from build123d import *

# Parameters (mm, degrees)
EXTRUDE_1_DEPTH = 20


with BuildPart() as part:
    # Эскиз1 → Бобышка-Вытянуть1 (new body)
    with BuildSketch(Plane.XY):
        Polygon((-9.845304567, -8.192930284), (40.154695433, -8.192930284), (40.154695433, -2.192930284), (19.154695433, -2.192930284), (19.154695433, -0.692930284), (23.154695433, 1.307069716), (23.154695433, 2.307069716), (19.154695433, 4.307069716), (11.154695433, 4.307069716), (7.154695433, 2.307069716), (7.154695433, 1.307069716), (11.154695433, -0.692930284), (11.154695433, -2.192930284), (-9.845304567, -2.192930284), align=None)
    extrude(amount=EXTRUDE_1_DEPTH)


solid = part.part
Read the model definition and answer for the solid it produces. Units are mm, in the model's axes. A direction names the side the tool comes from. Round coordinates to 2 decimals unless told otherwise and drop trailing zeros. Write each loop counter-clockwise with the first axis right and the second up, starting at its lowest first coordinate (ties: lowest second). Pieces come first, ordered by that corner, then holes.
1. Given pin 1 Ø1.2 at (y, z) = (-1.5, 10.5) entering from -X; pin 2 Ø6 at (x, z) = (28, 8) entering from +Y; pin 3 Ø0.8 at (y, z) = (1.5, 7.5) entering from -X; pin 4 Ø1.5 at (x, y) = (33, -4.5) entering from -Z, each flat-ended and moving along its own axis, determine where each tip first touches the part or whether it passes through.
2. Determine the mould class of faces 5 (the face through (19.155, -1, 10)), 6 (the face through (15, -8.193, 10)), 7 (the face through (21.127, 0.293, 9.86)), 8 (the face through (15, -3, 20)) for opening direction Y: pulls with the +Y half, pulls with the -Y half, needs draft (parallel to the pull), parting line crosses it, or undercut.
3. The part is cut by section D-D, the plane x = -5.5. Determine the outline of the cut face in (y, z), then the cut area to 3 significant figures.
4. Which of the six approach directions +Z, -Z, +X, -X, +Y, -Y give full straight-line access (tool end or side, diameter ignored) to faces 1 (the face through (7.155, 2, 10)), 2 (the face through (23.155, 2, 10)), 3 (the face through (30, -2.193, 10)), 4 (the face through (9.13, 0.32, 9.86))?
5. The part is cut by section A-A, the plane z = 15. Determine the outline of the cut face in (x, y), then the cut area to 3 significant figures.
6. The part is cut by section C-C, the plane y = -1.75. Determine the outline of the cut face in (x, z).
7. The part is cut by section B-B, the plane x = 8. Determine the outline of the cut face in (y, z), then the cut area to 3 significant figures.
8. Straight lines are drawn through the part: L1, parallel to Y at x = 1.5, z = 3.5; L2, parallel to X at y = 1.5, z = 15.75; L3, parallel to X at y = -0.75, z = 17.25. For each, find the intervals that lie inside material, in ascending order.
Values:
1. pin 1: stops at x = 11.15
1. pin 2: stops at y = -2.19
1. pin 3: stops at x = 7.15
1. pin 4: stops at z = 0
2. face 5: undercut
2. face 6: pulls with the -Y half
2. face 7: undercut
2. face 8: needs draft
3. outline: (-8.19, 0) - (-2.19, 0) - (-2.19, 20) - (-8.19, 20) - close
3. area: 120 mm2
4. face 1: +Z, -Z, -X, +Y
4. face 2: +Z, -Z, +X, +Y
4. face 3: +Z, -Z, +X
4. face 4: +Z, -Z, -X
5. outline: (-9.85, -8.19) - (40.15, -8.19) - (40.15, -2.19) - (19.15, -2.19) - (19.15, -0.69) - (23.15, 1.31) - (23.15, 2.31) - (19.15, 4.31) - (11.15, 4.31) - (7.15, 2.31) - (7.15, 1.31) - (11.15, -0.69) - (11.15, -2.19) - (-9.85, -2.19) - close
5. area: 376 mm2
6. outline: (11.15, 0) - (19.15, 0) - (19.15, 20) - (11.15, 20) - close
7. outline: (-8.19, 0) - (-2.19, 0) - (-2.19, 20) - (-8.19, 20) - close; (0.88, 0) - (2.73, 0) - (2.73, 20) - (0.88, 20) - close
7. area: 157 mm2
8. L1: y = -8.19 to -2.19
8. L2: x = 7.15 to 23.15
8. L3: x = 11.15 to 19.15
